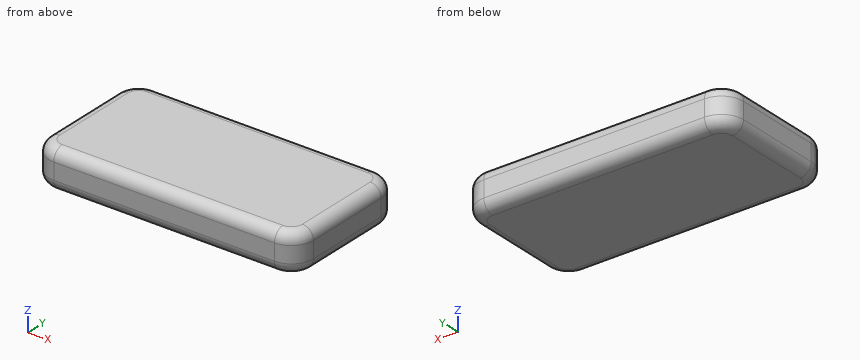
from build123d import *

# Parameters (mm, degrees)
F0_W     = 609.6
F0_H     = 304.8
F1_DEPTH = 88.9
F2_R     = 50.8
F3_R     = 25.4


with BuildPart() as f1:
    # F0 (on Top) → F1 (new body)
    with BuildSketch(Plane.XY):
        Rectangle(F0_W, F0_H)
    extrude(amount=F1_DEPTH)

    # F2
    f2_edges = [f1.edges().sort_by_distance(p)[0] for p in [
        (-304.8, 152.4, 44.45),
        (-304.8, -152.4, 44.45),
        (304.8, -152.4, 44.45),
        (304.8, 152.4, 44.45),
    ]]
    fillet(f2_edges, radius=F2_R)

    # F3
    f3_edges = [f1.edges().sort_by_distance(p)[0] for p in [
        (0, -152.4, 88.9),
        (0, 152.4, 88.9),
        (0, 152.4, 0),
    ]]
    fillet(f3_edges, radius=F3_R)


solid = f1.part
For this review, take the finished solid that the model builds, in its own axes (mm). Coordinates: 2 decimals unless noted, no trailing zeros. Order: outer loops, then holes, each group sorted by start corner. A loop starts at its lowest first (then second) coordinate and runs counter-clockwise, first axis right, second up. Notation, with made-up numbers: (68.25, 89) - (73.25, 89) arc R26 ccw to (73.25, 117) - close; hole circle Ø4 at (64.5, 64). An arc over 180 degrees is marked (long way). Answer as CSV lines item,"result". Start each with the question number.
1) Add section A-A (x = -241.5). State the section outline as (y, z) points.
2) To check wall thickness, follow line 1 along Z through (x, y) = (-142.5, -128); line 2 along Y through (x, z) = (-198, 23); line 3 along Y through (x, z) = (-177, 71). State the ranges of each line that lie inside material, in increasing order. Write a range as [from, to].
3) Insertion check: P1, Ø3, axis at y = -34.5, z = 19, coming from the -X side; P2, Ø5, axis at y = 65, z = 12, coming from the +X side; P3, Ø12, axis at y = -115, z = 9.5, coming from the +X side. Each pin has a flat end and moves straight along its axis. Give the tip position at first contact, or say it passes through.
Result:
1,outline,"(-152.4, 25.4) arc R25.4 ccw to (-127, 0) - (127, 0) arc R25.4 ccw to (152.4, 25.4) - (152.4, 63.5) arc R25.4 ccw to (127, 88.9) - (-127, 88.9) arc R25.4 ccw to (-152.4, 63.5) - close"
2,line 1,"[0.02, 88.88]"
2,line 2,"[-152.29, 152.29]"
2,line 3,"[-151.27, 151.27]"
3,P1,"x = -304.32"
3,P2,"x = 302.34"
3,P3,"x = 301.31"
